```python
from build123d import *

# Parameters (mm, degrees)
SKETCH1_W                      = 60
SKETCH1_H                      = 60
BOSS_EXTRUDE1_DEPTH            = 12
M12X1_75_TAPPED_HOLE1_D        = 10.2
CBORE_FOR_M8_SHCS1_D           = 9
CBORE_FOR_M8_SHCS1_CBORE_D     = 15
CBORE_FOR_M8_SHCS1_CBORE_DEPTH = 8
CHAMFER1_SIZE                  = 1


with BuildPart() as part:
    # Sketch1 → Boss-Extrude1 (new body)
    with BuildSketch(Plane.XY):
        Rectangle(SKETCH1_W, SKETCH1_H)
    extrude(amount=BOSS_EXTRUDE1_DEPTH)

    # M12x1.75 Tapped Hole1 (through all)
    with Locations(Plane.XY.offset(12)):
        with Locations((0, 0)):
            Hole(M12X1_75_TAPPED_HOLE1_D / 2)

    # CBORE for M8 SHCS1 (through all)
    with Locations(Plane.XY.offset(12)):
        with Locations((-15, 15), (15, 15), (15, -15), (-15, -15)):
            CounterBoreHole(CBORE_FOR_M8_SHCS1_D / 2, CBORE_FOR_M8_SHCS1_CBORE_D / 2, CBORE_FOR_M8_SHCS1_CBORE_DEPTH)

    # Chamfer1
    chamfer1_edges = [part.edges().sort_by_distance(p)[0] for p in [
        (30, -30, 6),
        (-30, -30, 6),
        (-30, 30, 6),
        (30, 30, 6),
    ]]
    chamfer(chamfer1_edges, length=CHAMFER1_SIZE)


solid = part.part
```
Geometry: final body of the model. Coordinates: model frame, mm. A direction names the side the tool comes from. Round coordinates to 2 decimals unless told otherwise and drop trailing zeros. Write each loop counter-clockwise with the first axis right and the second up, starting at its lowest first coordinate (ties: lowest second). Pieces come first, ordered by that corner, then holes. Notation, with made-up numbers: (8.25, -21) -> (59.25, -21) arc R22 cw to (59.25, 14) -> close; hole circle Ø2 at (31, 44). An arc over 180 degrees is marked (long way). Return JSON: item names as keys, results as strings.
Q1. Ray query, line 1 (Y direction, x = 15, z = 7); line 2 (Y direction, x = -15, z = 3.25); line 3 (X direction, y = 21.5, z = 6). Return the intervals inside material, ascending.
From the geometry:
{"line 1": "-30 to -22.5, -7.5 to 7.5, 22.5 to 30", "line 2": "-30 to -19.5, -10.5 to 10.5, 19.5 to 30", "line 3": "-30 to -18.74, -11.26 to 11.26, 18.74 to 30"}
Q2. Section A-A on y = 0. Return the cut outline in (x, z).
From the geometry:
{"outline": "(-30, 0) -> (-5.1, 0) -> (-5.1, 12) -> (-30, 12) -> close; (5.1, 0) -> (30, 0) -> (30, 12) -> (5.1, 12) -> close"}
Q3. Set-up query: faces 4 (the cylindrical face through (18.32, -11.96, 1.97)), 5 (the cylindrical face through (-22.493, 15.33, 8.056)). Return all of +Z, -Z, +X, -X, +Y, -Y with unobstructed straight access to the full face (end or side cutting, diameter ignored); none if empty.
From the geometry:
{"face 4": "+Z, -Z", "face 5": "+Z"}
Q4. Section D-D on y = -21. Return the cut outline in (x, z), and give its area (3 significant figures).
From the geometry:
{"outline": "(-30, 0) -> (30, 0) -> (30, 12) -> (19.5, 12) -> (19.5, 4) -> (10.5, 4) -> (10.5, 12) -> (-10.5, 12) -> (-10.5, 4) -> (-19.5, 4) -> (-19.5, 12) -> (-30, 12) -> close", "area": "576 mm2"}
Q5. Mould query, pull axis Y, two halves, no side actions, for faces 1 (the flat face through (30, 0, 6)), 2 (the cylindrical face through (-14.41, 19.46, 1.97)), 3 (the flat face through (0, -30, 6)). Classes: +Y half, -Y half, draft (parallel to the pull), parting line (faces both ways), or undercut.
From the geometry:
{"face 1": "draft", "face 2": "undercut", "face 3": "-Y half"}
Q6. Section B-B on z = 8.5. Return the cut outline in (x, y), and give its area (3 significant figures).
From the geometry:
{"outline": "(-30, -29) -> (-29, -30) -> (29, -30) -> (30, -29) -> (30, 29) -> (29, 30) -> (-29, 30) -> (-30, 29) -> close; hole circle Ø15 at (-15, -15); hole circle Ø15 at (-15, 15); hole circle Ø10.2 at (0, 0); hole circle Ø15 at (15, -15); hole circle Ø15 at (15, 15)", "area": "2,810 mm2"}
Q7. Section C-C on x = -15. Return the cut outline in (y, z).
From the geometry:
{"outline": "(-30, 0) -> (-19.5, 0) -> (-19.5, 4) -> (-22.5, 4) -> (-22.5, 12) -> (-30, 12) -> close; (-10.5, 0) -> (10.5, 0) -> (10.5, 4) -> (7.5, 4) -> (7.5, 12) -> (-7.5, 12) -> (-7.5, 4) -> (-10.5, 4) -> close; (19.5, 0) -> (30, 0) -> (30, 12) -> (22.5, 12) -> (22.5, 4) -> (19.5, 4) -> close"}
Q8. First-contact query: pin 1 Ø4.5 at (x, y) = (-11.5, -12) entering from +Z. Flat tip, straight axial feed; report the tip coordinate or a pass-through.
From the geometry:
{"pin 1": "z = 4"}
